from build123d import *

# Parameters (mm, degrees)
ESQUISSE2_R        = 33
BOSS_EXTRU_1_DEPTH = 145
ESQUISSE4_R        = 33
BOSS_EXTRU_2_DEPTH = 45
BOSS_EXTRU_2_TAPER = 24
ESQUISSE5_R        = 15
BOSS_EXTRU_3_DEPTH = 5


with BuildPart() as part:
    # Esquisse2 → Boss.-Extru.1 (new body)
    with BuildSketch(Plane.XY):
        with Locations((41.050709504, 36.47878936)):
            Circle(ESQUISSE2_R)
    extrude(amount=BOSS_EXTRU_1_DEPTH)

    # Esquisse4 → Boss.-Extru.2 (add)
    with BuildSketch(Plane.XY.offset(145)):
        with Locations((41.050709504, 36.47878936)):
            Circle(ESQUISSE4_R)
    extrude(amount=BOSS_EXTRU_2_DEPTH, taper=BOSS_EXTRU_2_TAPER)

    # Esquisse5 → Boss.-Extru.3 (add)
    with BuildSketch(Plane.XY.offset(190)):
        with Locations((41.050709504, 36.47878936)):
            Circle(ESQUISSE5_R)
    extrude(amount=BOSS_EXTRU_3_DEPTH)


solid = part.part
Could you check a few things on this model? Use its own coordinates, in mm. A direction names the side the tool comes from. Round coordinates to 2 decimals unless told otherwise and drop trailing zeros. Write each loop counter-clockwise with the first axis right and the second up, starting at its lowest first coordinate (ties: lowest second). Pieces come first, ordered by that corner, then holes. Notation, with made-up numbers: (89, 43) - (147, 43) arc R22 cw to (147, 66) - close; hole circle Ø4 at (-33, -34). An arc over 180 degrees is marked (long way). Use a Markdown table: item, result.
Q1. For pin 1 (1 mm diameter, centred on x = 27.5, z = 63, fed in from -Y); pin 2 (4 mm diameter, centred on y = 59, z = 30.5, fed in from +X); pin 3 (1 mm diameter, centred on x = 22.5, y = 25.5, fed in from +Z), each with a flat end and sliding along its axis, tell me the tip position at first contact or that it passes through.
Output values:
| item | result |
|---|---|
| pin 1 | y = 6.17 |
| pin 2 | x = 66.89 |
| pin 3 | z = 171.83 |
Q2. I want a section at A-A (z = 96.5). List the corners of the cut face in (x, y) for me, plus the area to 3 significant figures.
Output values:
| item | result |
|---|---|
| outline | circle Ø66 at (41.05, 36.48) |
| area | 3,420 mm2 |
Q3. Please list where these lines run through material, in increasing order: L1, parallel to Y at x = 41, z = 93.5; L2, parallel to X at y = 37, z = 38; L3, parallel to Z at x = 71.5, y = 32.
Output values:
| item | result |
|---|---|
| L1 | 3.48 to 69.48 |
| L2 | 8.05 to 74.05 |
| L3 | 0 to 149.99 |
Q4. I want a section at B-B (z = 176). List the corners of the cut face in (x, y) for me.
Output values:
| item | result |
|---|---|
| outline | circle Ø38.4 at (41.05, 36.48) |
Q5. For faces 4 (the flat face through (41, 37, 195)), 5 (the cylindrical face through (49.11, 49.13, 192.46)), which set-ups out of +Z, -Z, +X, -X, +Y, -Y let a thin tool reach every point of the face, with its end or its side?
Output values:
| item | result |
|---|---|
| face 4 | +Z, +X, -X, +Y, -Y |
| face 5 | +Z |
Q6. Thinking about a two-plate mould opening in Z: for faces 1 (the flat face through (41, 37, 0)), 2 (the cylindrical face through (16.728, 58.782, 71.485)), 3 (the flat face through (34, 48, 190)), which applies, released by +Z, released by -Z, zero draft, split by the parting line, or undercut?
Output values:
| item | result |
|---|---|
| face 1 | released by -Z |
| face 2 | zero draft |
| face 3 | undercut |
